Source: CAD feature listing. Evaluate the final solid. Frame: model axes, mm. A direction names the side the tool comes from. Round coordinates to 2 decimals unless told otherwise and drop trailing zeros. Loops run counter-clockwise (first coordinate to the right, second up) from the corner with the lowest first, then second, coordinate; pieces in that order, holes last. Notation, with made-up numbers: (59.5, 86) - (101.5, 86) arc R29 ccw to (101.5, 112) - close; hole circle Ø1 at (53, 72). An arc over 180 degrees is marked (long way). Write item = value, one per line. Start each with the question number.
from build123d import *

# Parameters (mm, degrees)
SKETCH_1_R                = 36.25
EXTRUDE_1_DEPTH           = 10
SKETCH_2_W                = 25
SKETCH_2_H                = 20.25
CUT_EXTRUDE_1_DEPTH       = 4.5
SKETCH_3_W                = 23.75
SKETCH_3_H                = 48.75
CUT_EXTRUDE_2_DEPTH       = 4.5
SKETCH_4_R                = 10
EXTRUDE_2_DEPTH           = 4.5
SKETCH_5_R                = 10
EXTRUDE_3_DEPTH           = 4.5
SKETCH_6_W                = 32
SKETCH_6_H                = 31.5
EXTRUDE_4_DEPTH           = 4.5
SKETCH_7_R                = 36.25
CUT_EXTRUDE_3_DEPTH       = 5.5
SKETCH_8_W                = 23.75
SKETCH_8_H                = 19.25
EXTRUDE_5_DEPTH           = 11
SKETCH_9_OUTSIDE_W        = 95.24
SKETCH_9_OUTSIDE_H        = 95.24
SKETCH_9_OUTSIDE_R        = 36.25
CUT_EXTRUDE_4_DEPTH       = 11
HOLE_WIZARD_1_D           = 1.6
HOLE_WIZARD_1_DEPTH       = 100
HOLE_WIZARD_1_CBORE_D     = 3.2
HOLE_WIZARD_1_CBORE_DEPTH = 14.1
HOLE_WIZARD_2_D           = 1.6
HOLE_WIZARD_2_DEPTH       = 100
HOLE_WIZARD_2_CBORE_D     = 3.2
HOLE_WIZARD_2_CBORE_DEPTH = 3.1
FILLET_1_R                = 1
FILLET_2_R                = 1


with BuildPart() as part:
    # 草图1 → 凸台-拉伸1 (new body)
    with BuildSketch(Plane.XY):
        Circle(SKETCH_1_R)
    extrude(amount=EXTRUDE_1_DEPTH)

    # 草图2 → 切除-拉伸1 (cut)
    with BuildSketch(Plane.XY):
        with Locations((0, 26.125)):
            Rectangle(SKETCH_2_W, SKETCH_2_H)
    extrude(amount=CUT_EXTRUDE_1_DEPTH, mode=Mode.SUBTRACT)

    # 草图3 → 切除-拉伸2 (cut)
    with BuildSketch(Plane.XY):
        with Locations((-24.375, -11.875)):
            Rectangle(SKETCH_3_W, SKETCH_3_H)
        with Locations((24.375, -11.875)):
            Rectangle(SKETCH_3_W, SKETCH_3_H)
    extrude(amount=CUT_EXTRUDE_2_DEPTH, mode=Mode.SUBTRACT)

    # 草图4 → 凸台-拉伸2 (add)
    with BuildSketch(Plane.XY):
        with Locations((-6, -19)):
            Circle(SKETCH_4_R)
    extrude(amount=EXTRUDE_2_DEPTH)

    # 草图5 → 凸台-拉伸3 (add)
    with BuildSketch(Plane.XY):
        with Locations((6, -19)):
            Circle(SKETCH_5_R)
    extrude(amount=EXTRUDE_3_DEPTH)

    # 草图6 → 凸台-拉伸4 (add)
    with BuildSketch(Plane.XY):
        with Locations((0, -3.25)):
            Rectangle(SKETCH_6_W, SKETCH_6_H)
    extrude(amount=EXTRUDE_4_DEPTH)

    # 草图7 → 切除-拉伸3 (cut)
    with BuildSketch(Plane(origin=(0, 0, 4.5), x_dir=(-1, 0, 0), z_dir=(0, 0, -1))):
        Circle(SKETCH_7_R)
    extrude(amount=-CUT_EXTRUDE_3_DEPTH, mode=Mode.SUBTRACT)

    # 草图8 → 凸台-拉伸5 (add)
    with BuildSketch(Plane.XY):
        with Locations((-24.375, 26.625)):
            Rectangle(SKETCH_8_W, SKETCH_8_H)
        with Locations((24.375, 26.625)):
            Rectangle(SKETCH_8_W, SKETCH_8_H)
    extrude(amount=-EXTRUDE_5_DEPTH)

    # 草图9 outside → 切除-拉伸4 (cut)
    with BuildSketch(Plane.XY):
        Rectangle(SKETCH_9_OUTSIDE_W, SKETCH_9_OUTSIDE_H)
        Circle(SKETCH_9_OUTSIDE_R, mode=Mode.SUBTRACT)
    extrude(amount=-CUT_EXTRUDE_4_DEPTH, mode=Mode.SUBTRACT)

    # 孔1
    with Locations(Plane.XY.offset(4.5)):
        with Locations((-21, 21), (21, 21)):
            CounterBoreHole(HOLE_WIZARD_1_D / 2, HOLE_WIZARD_1_CBORE_D / 2, HOLE_WIZARD_1_CBORE_DEPTH, depth=HOLE_WIZARD_1_DEPTH)

    # 孔2
    with Locations(Plane.XY.offset(4.5)):
        with Locations((0, -30)):
            CounterBoreHole(HOLE_WIZARD_2_D / 2, HOLE_WIZARD_2_CBORE_D / 2, HOLE_WIZARD_2_CBORE_DEPTH, depth=HOLE_WIZARD_2_DEPTH)

    # 圆角1
    fillet_1_edges = [part.edges().sort_by_distance(p)[0] for p in [
        (-16, 12.5, 2.25),
        (16, 12.5, 2.25),
        (12.5, 16, 2.25),
        (-12.5, 34.026643972, -3.25),
        (-12.5, 16, 2.25),
        (12.5, 34.026643972, -3.25),
        (-12.5, -34.026643972, 2.25),
        (-34.026643972, 12.5, 2.25),
        (12.5, -34.026643972, 2.25),
        (34.026643972, 12.5, 2.25),
        (-12.5, -26.599342077, 2.25),
        (12.5, -26.599342077, 2.25),
    ]]
    fillet(fillet_1_edges, radius=FILLET_1_R)

    # 圆角2
    fillet_2_edges = [part.edges().sort_by_distance(p)[0] for p in [
        (-16.292893219, 12.207106781, 4.5),
        (-24.78122001, 12.5, 4.5),
        (-33.393998413, 12.94456266, 4.5),
        (0, -36.25, 4.5),
        (-12.94456266, 33.393998413, 4.5),
        (-12.5, 24.78122001, 4.5),
        (-12.207106781, 16.292893219, 4.5),
        (0, 16, 4.5),
        (12.207106781, 16.292893219, 4.5),
        (12.5, 24.78122001, 4.5),
        (12.94456266, 33.393998413, 4.5),
        (33.393998413, 12.94456266, 4.5),
        (24.78122001, 12.5, 4.5),
        (16.292893219, 12.207106781, 4.5),
        (16, -3.75, 4.5),
        (15.170109546, -22.988620176, 4.5),
        (12.582989045, -26.647876452, 4.5),
        (12.5, -30.184045242, 4.5),
        (12.314322152, -33.90176517, 4.5),
        (-12.314322152, -33.90176517, 4.5),
        (-12.5, -30.184045242, 4.5),
        (-12.582989045, -26.647876452, 4.5),
        (-15.170109546, -22.988620176, 4.5),
        (-16, -3.75, 4.5),
    ]]
    fillet(fillet_2_edges, radius=FILLET_2_R)


solid = part.part
(1) Cut plane D-D (y = -17). Output: boundary loops of the cut face in (x, z).
(2) Cut plane B-B (y = -30). Output: boundary loops of the cut face in (x, z), and give its area (3 significant figures).
(3) Cut plane A-A (z = -7.5). Output: boundary loops of the cut face in (x, y), and give its area (3 significant figures).
(4) Material intervals for line 1 along Y through (x, z) = (-21, -10.1); line 2 along Y through (x, z) = (-21, -5.25); line 3 along Z through (x, y) = (-6, -27.5), sorted ascending. Write a range as from..to.
(5) Access query for faces 1 (the face through (16, -4, 2)), 2 (the face through (-25, 12.5, 2)), 3 (the face through (22, 17, -5)), 4 (the face through (-12.5, 25, -4)), 5 (the face through (-22, 21, -9.6)). Directions: +Z, -Z, +X, -X, +Y, -Y. A direction counts if a zero-diameter tool reaches every point of the face in a straight line with its end or side. Return the directions, or none.
(6) Mould query, pull axis Y, two halves, no side actions, for faces 6 (the face through (-0.17, -36.25, 1.73)), 7 (the face through (0, 16, 2)), 8 (the face through (-21.37, 20.29, -10.31)), 9 (the face through (-16, -4, 2)). Classes: +Y half, -Y half, draft (parallel to the pull), parting line (faces both ways), or undercut.
(7) Pin query (flat end, axial travel): P1, Ø1, axis at x = 3, z = 1.5, coming from the +Y side; P2, Ø1, axis at x = 20.5, z = -6, coming from the +Y side; P3, Ø1.3, axis at x = -21, y = 21, coming from the +Z side; P4, Ø1.8, axis at y = -31.5, z = 1.5, coming from the -X side. Return the tip coordinate at first contact, or that it passes through.
(8) Cut plane C-C (x = 0). Output: boundary loops of the cut face in (y, z), and give its area (3 significant figures).
Solution:
q1.outline = (-16, 0) - (16, 0) - (16, 3.5) arc R1 ccw to (15, 4.5) - (-15, 4.5) arc R1 ccw to (-16, 3.5) - close
q2.outline = (-12.5, 0) - (-0.8, 0) - (-0.8, 1.4) - (-1.6, 1.4) - (-1.6, 4.5) - (-11.5, 4.5) arc R1 ccw to (-12.5, 3.5) - close; (0.8, 0) - (12.5, 0) - (12.5, 3.5) arc R1 ccw to (11.5, 4.5) - (1.6, 4.5) - (1.6, 1.4) - (0.8, 1.4) - close
q2.area = 99.9 mm^2
q3.outline = (-32.02, 17) - (-12.5, 17) - (-12.5, 32.56) arc R1 ccw to (-13.88, 33.49) arc R36.25 ccw to start; (12.5, 17) - (32.02, 17) arc R36.25 ccw to (13.88, 33.49) arc R1 ccw to (12.5, 32.56) - close; hole circle Ø3.2 at (-21, 21); hole circle Ø3.2 at (21, 21)
q3.area = 398 mm^2
q4.line_1 = 17..20.2, 21.8..29.55
q4.line_2 = 17..19.4, 22.6..29.55
q4.line_3 = 0..4.5
q5.face_1 = +Z, -Z, +X, -Y
q5.face_2 = +Z, -Z, -X, -Y
q5.face_3 = -Z, +X, -X, -Y
q5.face_4 = +Z, -Z, +Y
q5.face_5 = +Z
q6.face_6 = -Y half
q6.face_7 = +Y half
q6.face_8 = undercut
q6.face_9 = draft
q7.P1 = 16
q7.P2 = 30.23
q7.P3 = through
q7.P4 = -12.5
q8.outline = (-36.25, 0) - (-30.8, 0) - (-30.8, 1.4) - (-31.6, 1.4) - (-31.6, 4.5) - (-35.25, 4.5) arc R1 ccw to (-36.25, 3.5) - close; (-29.2, 0) - (16, 0) - (16, 3.5) arc R1 ccw to (15, 4.5) - (-28.4, 4.5) - (-28.4, 1.4) - (-29.2, 1.4) - close
q8.area = 223 mm^2
